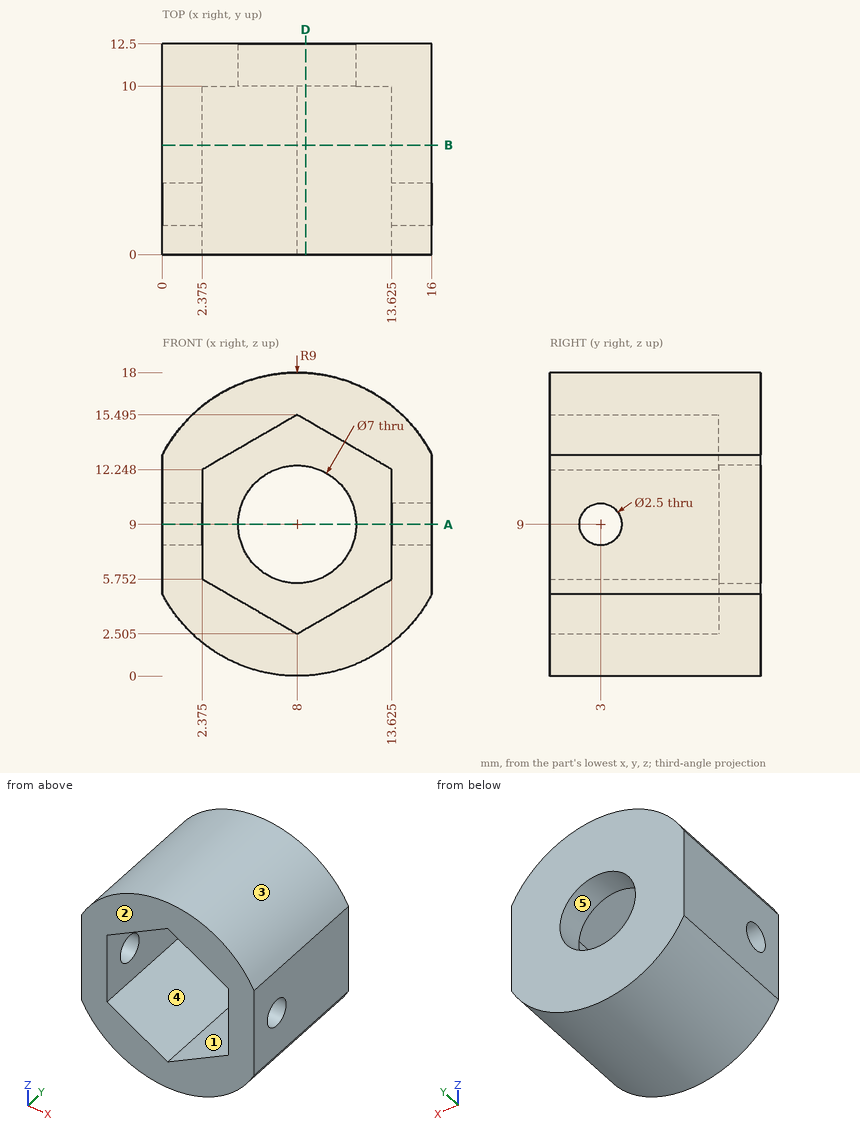
Can you work these out from the drawing? Everything is in mm from the part's minimum corner. A direction names the side the tool comes from. Give positions to 0.01 mm unless a question says otherwise; leave off trailing zeros. Loops run counter-clockwise (first coordinate to the right, second up) from the corner with the lowest first, then second, coordinate; pieces in that order, holes last. Notation, with made-up numbers: M 43.5,38 L 77.5,38 A19 ccw 77.5,57 Z; hole C 73.5,33 d10. An arc over 180 degrees is marked long. Use CSV: the item, a comma, the result in double quotes. Start each with the question number.
1. Imagine slicing it at B-B, the plane y = 6.5. Write out the boundary of the cut face in (x, z) (1 decimal), plus the area to 3 significant figures.
2. If I drill on L1, parallel to X at y = 8, z = 7.5 (1 decimal); L2, parallel to X at y = 10.65, z = 9; L3, parallel to Y at x = 8.25, z = 15, over which ranges is the centre line in solid material (lowest first)?
3. On a 3-axis mill with a long thin cutter (end or side, diameter ignored), from which of +Z, -Z, +X, -X, +Y, -Y can I reach the whole of each face in a straight line? I mean the marked faces 4 and 5. Say none if no direction works.
4. For P1, Ø2, axis at y = 3, z = 9, coming from the -X side; P2, Ø1, axis at x = 2, y = 7.5, coming from the +Z side (1 decimal); P3, Ø1.5, axis at x = 9.5, y = 8, coming from the +Z side, each with a flat end and sliding along its axis, tell me the tip position at first contact or that it passes through.
5. Imagine slicing it at D-D, the plane x = 8.5. Write out the boundary of the cut face in (y, z).
6. If we mould it in two halves opening along X, with no side actions, what happens to the marked faces 1, 2 and 3? For each: released by +X, released by -X, zero draft, split by the parting line, or undercut.
7. Imagine slicing it at A-A, the plane z = 9. Count the separate pieces of the cut face and the enclosed holes in it.
Response values:
1,outline,"M 0,4.9 A9 ccw 16,4.9 L 16,13.1 A9 ccw 0,13.1 Z; hole M 2.4,5.8 L 8,2.5 L 13.6,5.8 L 13.6,12.2 L 8,15.5 L 2.4,12.2 Z"
1,area,"134 mm^2"
2,L1,"0 to 2.4, 13.6 to 16"
2,L2,"0 to 4.5, 11.5 to 16"
2,L3,"10 to 12.5"
3,face 4,"-Y"
3,face 5,"+Y, -Y"
4,P1,"through"
4,P2,"z = 16.1"
4,P3,"z = 17.97"
5,outline,"M 0,0.01 L 12.5,0.01 L 12.5,5.54 L 10,5.54 L 10,2.79 L 0,2.79 Z; M 0,15.21 L 10,15.21 L 10,12.46 L 12.5,12.46 L 12.5,17.99 L 0,17.99 Z"
6,face 1,"undercut"
6,face 2,"zero draft"
6,face 3,"split by the parting line"
7,separate pieces,"4"
7,enclosed holes,"0"
